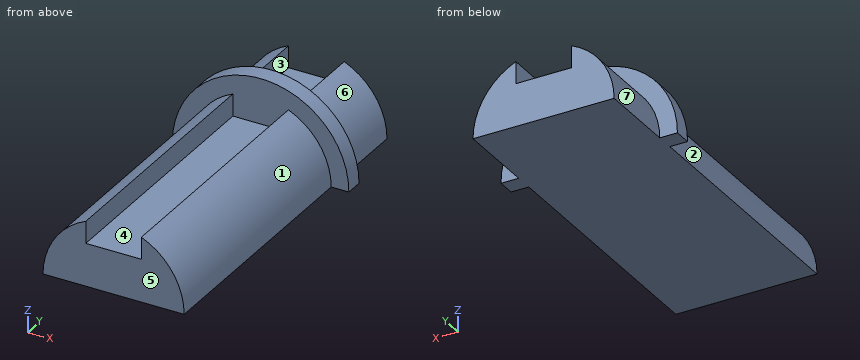
Autodesk Inventor part; units mm, degrees
ref_plane "YZ Plane" through (0, 0, 0) normal (1, 0, 0) x (0, 1, 0)
ref_plane "XZ Plane" through (0, 0, 0) normal (0, 1, 0) x (-1, 0, 0)
ref_plane "XY Plane" through (0, 0, 0) normal (0, 0, 1) x (1, 0, 0)
sketch "Sketch1" plane through (0, 0, 0) normal (0, 1, 0) x (-1, 0, 0)
  circle A0 centre (0, 0) radius 4
  line L0 (-1.575, 5.575) -> (1.575, 5.575)
  line L1 (1.575, 5.575) -> (1.575, 2.425)
  line L2 (1.575, 2.425) -> (-1.575, 2.425)
  line L3 (-1.575, 2.425) -> (-1.575, 5.575)
  line L4 (-1.575, 5.575) -> (1.575, 2.425) construction
  line L5 (1.575, 5.575) -> (-1.575, 2.425) construction
  line L6 (-1.575, -2.425) -> (1.575, -2.425)
  line L7 (1.575, -2.425) -> (1.575, -5.575)
  line L8 (1.575, -5.575) -> (-1.575, -5.575)
  line L9 (-1.575, -5.575) -> (-1.575, -2.425)
  line L10 (-1.575, -2.425) -> (1.575, -5.575) construction
  line L11 (1.575, -2.425) -> (-1.575, -5.575) construction
  point P0 (0, 0)
  point P1 (0, 4)
  point P2 (0, -4)
  point P3 (-1.575, 3.6769)
  point P4 (-1.575, -3.6769)
  point P5 (1.575, -3.6769)
  point P6 (1.575, 3.6769)
  dimension "d0" = 8
  dimension "d10" = 3.15
  dimension "d11" = 3.15
  dimension "d12" = 3.15
  dimension "d13" = 3.15
extrude "Extrusion1" add sketch "Sketch1" along normal blind 5 and the other way blind 15 contours A0 L7 L6 L9 L3 L2 L1
sketch "Sketch2" plane through (0, 0, 0) normal (0, 1, 0) x (-1, 0, 0)
  circle A0 centre (0, 0) radius 5
  dimension "d3" = 10
extrude "Extrusion2" add sketch "Sketch2" along normal mid plane 1
sketch "Sketch3" plane through (0, 5, 0) normal (0, 1, 0) x (0, 0, 1)
  line L0 (0, -14) -> (-10, -14)
  line L1 (-10, -14) -> (-10, 12)
  line L2 (-10, 12) -> (0, 12)
  line L3 (0, 12) -> (0, -14)
  point P0 (0, 0)
extrude "Extrusion3" cut sketch "Sketch3" against normal blind 22
properties part number "halfAxel"
CAD build for the part. Positions are in the model's coordinates, mm. Face numbers are marked on the shaded views. A direction names the side the tool comes from. Round coordinates to 2 decimals unless told otherwise and drop trailing zeros. Order: outer loops, then holes, each group sorted by start corner. A loop starts at its lowest first (then second) coordinate and runs counter-clockwise, first axis right, second up. Notation, with made-up numbers: (26, -2.75) - (57, -2.75) arc R13 ccw to (57, 1.25) - close; hole circle Ø1 at (59.5, -1). An arc over 180 degrees is marked (long way). Answer in a Markdown table with one row per item. Add a question column.
(1) Drop flat-ended pins along their axis: pin 1 Ø2.5 at (x, y) = (-0.5, 3.5) entering from +Z; pin 2 Ø0.6 at (y, z) = (-8.5, 3) entering from +X; pin 3 Ø1 at (y, z) = (2, 3) entering from -X; pin 4 Ø1 at (x, y) = (-1, -10) entering from -Z. Give the stop position or say it passes through.
(2) Band-saw the part on B-B on y = -4.25. List the corners of the cut face in (x, z) (3 decimals), and give its area (3 significant figures).
(3) Mould opens along X. For the marked faces 1, 2 and 3 say: +X half, -X half, draft (parallel to the pull), parting line (faces both ways), or undercut.
(4) 3-axis set-ups, long thin cutter, end or side, ignore diameter. For the marked faces 4, 5, 6 and 7: which of +Z, -Z, +X, -X, +Y, -Y reach the whole face in a straight line?
(5) Band-saw the part on A-A on x = 0. List the corners of the cut face in (y, z) (3 decimals).
(6) Band-saw the part on D-D on x = -1.25. List the corners of the cut face in (y, z) (3 decimals).
(7) Band-saw the part on C-C on z = 0.6. List the corners of the cut face in (x, y), and give its area (3 significant figures).
(8) Probe L1, parallel to Z at x = 1, y = -1.5 (3 decimals); L2, parallel to Y at x = -1.5, z = 2.55; L3, parallel to X at y = 1, z = 3 (3 decimals). List the from-to ranges inside material, lowest first. Write a range as [from, to].
Data:
| question | item | result |
|---|---|---|
| 1 | pin 1 | stops at z = 3.68 |
| 1 | pin 2 | stops at x = 2.95 |
| 1 | pin 3 | stops at x = -3.12 |
| 1 | pin 4 | stops at z = 0 |
| 2 | outline | (-4, 0) - (4, 0) arc R4 ccw to (1.575, 3.677) - (1.575, 2.425) - (-1.575, 2.425) - (-1.575, 3.677) arc R4 ccw to start |
| 2 | area | 20.5 mm^2 |
| 3 | face 1 | +X half |
| 3 | face 2 | -X half |
| 3 | face 3 | undercut |
| 4 | face 4 | +Z, -Y |
| 4 | face 5 | +Z, -Z, +X, -X, -Y |
| 4 | face 6 | +Z, +X, +Y |
| 4 | face 7 | +Z, -X, +Y |
| 5 | outline | (-15, 0) - (5, 0) - (5, 2.425) - (0.5, 2.425) - (0.5, 5) - (-0.5, 5) - (-0.5, 2.425) - (-15, 2.425) - close |
| 6 | outline | (-15, 0) - (5, 0) - (5, 2.425) - (0.5, 2.425) - (0.5, 4.841) - (-0.5, 4.841) - (-0.5, 2.425) - (-15, 2.425) - close |
| 7 | outline | (-4.96, -0.5) - (-3.95, -0.5) - (-3.95, -15) - (3.95, -15) - (3.95, -0.5) - (4.96, -0.5) - (4.96, 0.5) - (3.95, 0.5) - (3.95, 5) - (-3.95, 5) - (-3.95, 0.5) - (-4.96, 0.5) - close |
| 7 | area | 160 mm^2 |
| 8 | L1 | z = [0, 2.425] |
| 8 | L2 | y = [-0.5, 0.5] |
| 8 | L3 | x = [-2.646, -1.575], [1.575, 2.646] |
